from build123d import *

# Parameters (mm, degrees)
F0_R     = 19.6
F0_R_2   = 8.55
F1_DEPTH = 5.2
F3_DEPTH = 9.2
F4_DEPTH = 5.201


with BuildPart() as f1:
    # F0 (on Top) → F1 (new body)
    with BuildSketch(Plane.XY):
        Circle(F0_R)
        Circle(F0_R_2, mode=Mode.SUBTRACT)
    extrude(amount=F1_DEPTH)

    # F2 (on face) → F3 (join)
    with BuildSketch(Plane.XY.offset(5.2)):
        with BuildLine():
            ThreePointArc((-12.5561737803, -15.05), (0, -19.6), (12.5561737803, -15.05))
            Line((12.5561737803, -15.05), (-12.5561737803, -15.05))
        make_face()
        with BuildLine():
            Line((-12.5561737803, 15.05), (12.5561737803, 15.05))
            ThreePointArc((12.5561737803, 15.05), (0, 19.6), (-12.5561737803, 15.05))
        make_face()
    extrude(amount=F3_DEPTH)

    # F2 (on face) → F4 (cut, through all)
    with BuildSketch(Plane.XY.offset(5.2)):
        with BuildLine():
            ThreePointArc((-15.05, 12.5561737803), (-19.6, 0), (-15.05, -12.5561737803))
            Line((-15.05, -12.5561737803), (-15.05, 12.5561737803))
        make_face()
        with BuildLine():
            Line((15.05, 12.5561737803), (15.05, -12.5561737803))
            ThreePointArc((15.05, -12.5561737803), (18.4274252135, -6.6775744099), (19.6, 0))
            ThreePointArc((19.6, 0), (18.4274252135, 6.6775744099), (15.05, 12.5561737803))
        make_face()
    extrude(amount=-F4_DEPTH, mode=Mode.SUBTRACT)


solid = f1.part
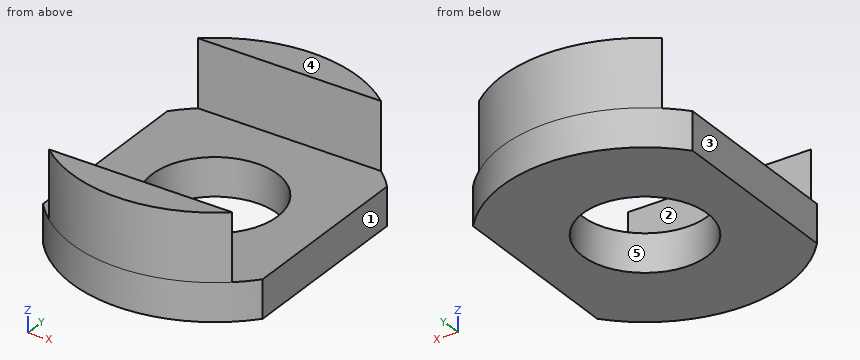
The listing builds one solid part. Answer for the finished solid, in the listing's coordinates (mm). Face numbers are marked on the shaded views. A direction names the side the tool comes from. Give positions to 0.01 mm unless a question says otherwise; leave off trailing zeros. Order: outer loops, then holes, each group sorted by start corner. A loop starts at its lowest first (then second) coordinate and runs counter-clockwise, first axis right, second up. Notation, with made-up numbers: (-10.5, 73) - (13.5, 73) arc R20 ccw to (13.5, 78) - close; hole circle Ø5 at (-36.75, 19). An arc over 180 degrees is marked (long way). Use one line per item in the form item = value.
1) Find section B-B on y = 0. Determine the outline of the cut face in (x, z).
Verdict:
outline = (-15.05, 0) - (-8.55, 0) - (-8.55, 5.2) - (-15.05, 5.2) - close; (8.55, 0) - (15.05, 0) - (15.05, 5.2) - (8.55, 5.2) - close
2) Find section D-D on x = 9. Determine the outline of the cut face in (y, z), and give its area (3 significant figures).
Verdict:
outline = (-17.41, 0) - (17.41, 0) - (17.41, 14.4) - (15.05, 14.4) - (15.05, 5.2) - (-15.05, 5.2) - (-15.05, 14.4) - (-17.41, 14.4) - close
area = 225 mm^2
3) Consider probe 1 along Y at (x, z) = (0, 3.85); probe 2 along Z at (x, y) = (-11, 14); probe 3 along X at (y, z) = (2, 3.5). Determine where each line is inside the solid, lowest interval first. Write a range as [from, to].
Verdict:
probe_1 = [-19.6, -8.55], [8.55, 19.6]
probe_2 = [0, 5.2]
probe_3 = [-15.05, -8.31], [8.31, 15.05]
4) Find section C-C on z = 10.75. Determine the outline of the cut face in (x, y), and give its area (3 significant figures).
Verdict:
outline = (-12.56, -15.05) arc R19.6 ccw to (12.56, -15.05) - close; (-12.56, 15.05) - (12.56, 15.05) arc R19.6 ccw to start
area = 156 mm^2
5) For the marked faces 1 and 2, determine the directions among +Z, -Z, +X, -X, +Y, -Y from which every point of the face is accessible in a straight line to the end or side of a thin tool.
Verdict:
face_1 = +Z, -Z, +X, +Y, -Y
face_2 = +Z, +X, -X
6) Each of these flat-tipped pins is pushed along its axis until it touches: pin 1 (6 mm diameter, centred on x = -9.5, z = 4, fed in from +Y); pin 2 (4.5 mm diameter, centred on x = 5, z = 9, fed in from -Y); pin 3 (4.5 mm diameter, centred on x = -1.5, z = 11.5, fed in from +Y). Where does it stop, or does it pass through?
Verdict:
pin_1 = 18.49
pin_2 = -19.41
pin_3 = 19.6
7) The mould has two halves that part along X. Classify the marked faces 3, 4 and 5: released by +X, released by -X, zero draft, split by the parting line, or undercut.
Verdict:
face_3 = released by -X
face_4 = zero draft
face_5 = undercut
8) Find section A-A on x = 0. Determine the outline of the cut face in (y, z).
Verdict:
outline = (-19.6, 0) - (-8.55, 0) - (-8.55, 5.2) - (-15.05, 5.2) - (-15.05, 14.4) - (-19.6, 14.4) - close; (8.55, 0) - (19.6, 0) - (19.6, 14.4) - (15.05, 14.4) - (15.05, 5.2) - (8.55, 5.2) - close
